Autodesk Inventor part; units mm, degrees
ref_plane "YZ Plane" through (0, 0, 0) normal (1, 0, 0) x (0, 1, 0)
ref_plane "XZ Plane" through (0, 0, 0) normal (0, 1, 0) x (-1, 0, 0)
ref_plane "XY Plane" through (0, 0, 0) normal (0, 0, 1) x (1, 0, 0)
sketch "スケッチ1" plane through (0, 0, 0) normal (0, 0, 1) x (1, 0, 0)
  line L0 (0, 37.5) -> (0, -37.5)
  line L1 (0, -37.5) -> (4.7631, -37.5)
  line L2 (4.7631, -37.5) -> (4.7631, 37.5)
  line L3 (4.7631, 37.5) -> (0, 37.5)
  point P0 (0, 0)
  point P1 (0, 0)
  dimension "d0" = 75
  dimension "d1" = 4.7631
revolve "回転1" add sketch "スケッチ1" angle 360 about axis through (0, 37.5, 0) along (0, -1, 0)
sketch "スケッチ2" plane through (0, 37.5, 0) normal (0, 1, 0) x (1, 0, 0)
  line L0 (3.1754, 0) -> (1.5877, -2.75)
  line L1 (1.5877, -2.75) -> (-1.5877, -2.75)
  line L2 (-1.5877, -2.75) -> (-3.1754, 0)
  line L3 (-3.1754, 0) -> (-1.5877, 2.75)
  line L4 (-1.5877, 2.75) -> (1.5877, 2.75)
  line L5 (1.5877, 2.75) -> (3.1754, 0)
  circle A0 centre (0, 0) radius 4.7631
  point P0 (0, 0)
  dimension "d3" = 5.5
extrude "押し出し1" cut sketch "スケッチ2" against normal through all
hole "穴1" at (0, 37.5, 0) direction (0, -1, 0) diameter 2.459 depth 6
sketch "スケッチ3" plane through (-1.5877, -37.5, 2.75) normal (0, -1, 0) x (1, 0, 0)
  point P0 (1.5877, -2.75)
  point P1 (1.5877, -2.75)
hole "穴2" at (0, -37.5, 0) direction (0, 1, 0) diameter 2.459 depth 6
properties part number "ASU-370H" material "アルミニウム 2014-T4"
The model under review builds one solid part; all positions refer to its coordinate system, in mm. A direction names the side the tool comes from. Give positions to 0.01 mm unless a question says otherwise; leave off trailing zeros. Write each loop counter-clockwise with the first axis right and the second up, starting at its lowest first coordinate (ties: lowest second). Pieces come first, ordered by that corner, then holes.
(1) Consider section B-B, the plane x = 0. Give the boundary of the cut face in (y, z), and give its area (3 significant figures).
(2) To check wall thickness, follow L1, parallel to X at y = 36, z = 0; L2, parallel to Z at x = 0, y = -35.1; L3, parallel to Z at x = -2.25, y = 21.5. State the ranges of each line that lie inside material, in increasing order.
(3) Consider section A-A, the plane y = -21. Give the boundary of the cut face in (x, z).
(4) The part is to be moulded in two halves that separate along X. For faces 4 (the cylindrical face through (0.748, -34.458, 0.976)), 5 (the flat face through (2.39, 0.52, 1.36)), 6 (the flat face through (0, 1, -2.75)), say which applies: released by +X, released by -X, zero draft, split by the parting line, or undercut.
(5) For P1, Ø2, axis at x = 0, z = 0, coming from the -Y side; P2, Ø0.7, axis at x = 0, z = 0.5, coming from the +Y side; P3, Ø1.5, axis at y = -1.5, z = 0.5, coming from the +X side, all flat-tipped, find the tip position at first contact; note any pin that passes through.
(6) Tool access review of faces 1 (the cylindrical face through (0.748, 34.458, -0.976)), 2 (the flat face through (1.4, 37.5, 0)), 3 (the flat face through (0, -31.5, 0)): name each direction out of +Z, -Z, +X, -X, +Y, -Y from which nothing blocks a thin tool from reaching the whole face with its end or side.
Returned:
1. outline: (-37.5, -2.75) - (37.5, -2.75) - (37.5, -1.23) - (31.5, -1.23) - (31.5, 1.23) - (37.5, 1.23) - (37.5, 2.75) - (-37.5, 2.75) - (-37.5, 1.23) - (-31.5, 1.23) - (-31.5, -1.23) - (-37.5, -1.23) - close
1. area: 383 mm2
2. L1: x = -3.18 to -1.23, 1.23 to 3.18
2. L2: z = -2.75 to -1.23, 1.23 to 2.75
2. L3: z = -1.6 to 1.6
3. outline: (-3.18, 0) - (-1.59, -2.75) - (1.59, -2.75) - (3.18, 0) - (1.59, 2.75) - (-1.59, 2.75) - close
4. face 4: undercut
4. face 5: released by +X
4. face 6: zero draft
5. P1: stops at y = -31.5
5. P2: stops at y = 31.5
5. P3: stops at x = 3.18
6. face 1: +Y
6. face 2: +Z, -Z, +X, -X, +Y
6. face 3: -Y
